```python
from build123d import *

# Parameters (mm, degrees)
BOSS_EXTRUDE1_DEPTH = 105
CUT_EXTRUDE1_REACH  = 238.485
SKETCH2_W           = 65
SKETCH2_H           = 15
CUT_EXTRUDE12_DEPTH = 281.35970199
CUT_EXTRUDE14_REACH = 239.237
FILLET1_R           = 10
FILLET2_R           = 10
FILLET3_R           = 10
FILLET4_R           = 2
CUT_EXTRUDE15_REACH = 239.237
SKETCH13_R          = 5
FILLET5_R           = 10


with BuildPart() as part:
    # Sketch1 → Boss-Extrude1 (new body)
    with BuildSketch(Plane.XY):
        Polygon((-125, -1.25), (125, -1.25), (126.885753532, -1.25), (146.885753532, 68.75), (200, 68.75), (200, 71.25), (145, 71.25), (125, 1.25), (-125, 1.25), align=None)
    extrude(amount=BOSS_EXTRUDE1_DEPTH)

    # Sketch2 → Cut-Extrude1 (cut, up to next)
    with BuildSketch(Plane(origin=(0, 1.25, 0), x_dir=(1, 0, 0), z_dir=(0, 1, 0)), mode=Mode.PRIVATE) as cut_extrude1_sk1:
        with Locations((-92.5, -52.5)):
            Rectangle(SKETCH2_W, SKETCH2_H)
    cut_extrude1_tool1 = extrude(cut_extrude1_sk1.sketch, amount=-CUT_EXTRUDE1_REACH, mode=Mode.PRIVATE) & part.part
    add(cut_extrude1_tool1.solids().sort_by_distance((-92.5, 1.25, 52.5))[0], mode=Mode.SUBTRACT)

    # Sketch11 → Cut-Extrude12 (cut, through all)
    with BuildSketch(Plane(origin=(125, 0, 0), x_dir=(0, 0, -1), z_dir=(1, 0, 0))):
        Polygon((0, 71.25), (0, 1.25), (-32.5, 68.75), (-32.5, 71.25), align=None)
        Polygon((-72.5, 68.75), (-72.5, 71.25), (-105, 71.25), (-105, 1.25), align=None)
    extrude(amount=CUT_EXTRUDE12_DEPTH, mode=Mode.SUBTRACT)

    # Sketch12 → Cut-Extrude14 (cut, up to next)
    with BuildSketch(Plane(origin=(0, 71.25, 0), x_dir=(1, 0, 0), z_dir=(0, 1, 0)), mode=Mode.PRIVATE) as cut_extrude14_sk1:
        Polygon((200, -62.5), (147.5, -72.5), (200, -72.5), align=None)
    cut_extrude14_tool1 = extrude(cut_extrude14_sk1.sketch, amount=-CUT_EXTRUDE14_REACH, mode=Mode.PRIVATE) & part.part
    # Sketch12 → Cut-Extrude14 (cut, up to next)
    with BuildSketch(Plane(origin=(0, 71.25, 0), x_dir=(1, 0, 0), z_dir=(0, 1, 0)), mode=Mode.PRIVATE) as cut_extrude14_sk2:
        Polygon((200, -32.5), (147.5, -32.5), (200, -42.5), align=None)
    cut_extrude14_tool2 = extrude(cut_extrude14_sk2.sketch, amount=-CUT_EXTRUDE14_REACH, mode=Mode.PRIVATE) & part.part
    add(cut_extrude14_tool1.solids().sort_by_distance((182.5, 71.25, 69.166667))[0], mode=Mode.SUBTRACT)
    add(cut_extrude14_tool2.solids().sort_by_distance((182.5, 71.25, 35.833333))[0], mode=Mode.SUBTRACT)

    # Fillet1
    fillet1_edges = [part.edges().sort_by_distance(p)[0] for p in [
        (200, 70, 42.5),
        (200, 70, 62.5),
    ]]
    fillet(fillet1_edges, radius=FILLET1_R)

    # Fillet2
    # the kernel refuses this fillet: 10 mm, written as the material it adds along each edge
    with BuildSketch(Plane(origin=(146.885753532, 68.75, 32.5), x_dir=(1, 0, 0), z_dir=(0, 0, 1))) as fillet2_piece_1_section:
        with BuildLine():
            CenterArc((FILLET2_R * 0.754301412754, -FILLET2_R), FILLET2_R, 90, 74.054604099)
            Line((-FILLET2_R * 0.207222534886, -FILLET2_R * 0.725278872103), (0, 0))
            Line((0, 0), (FILLET2_R * 0.754301412754, 0))
        make_face()
    fillet2_piece_1 = extrude(amount=40, mode=Mode.PRIVATE)
    fillet2_piece_1 = split(fillet2_piece_1, bisect_by=Plane(origin=(151.701250416, 67.179105295, 33.300238174), z_dir=(-0.18711210788999527, 0, 0.9823385664224747)), keep=Keep.TOP, mode=Mode.PRIVATE)
    fillet2_piece_1 = split(fillet2_piece_1, bisect_by=Plane(origin=(151.701250416, 67.179105295, 71.699761826), z_dir=(-0.18711210788999538, 0, -0.9823385664224747)), keep=Keep.TOP, mode=Mode.PRIVATE)
    add(fillet2_piece_1)
    # the kernel refuses this fillet: 10 mm, written as the material it takes off along each edge
    with BuildSketch(Plane(origin=(145, 71.25, 13.642464681), x_dir=(-0.27472112789737757, -0.9615239476408233, 0), z_dir=(0, 0, 1))) as fillet2_2_piece_1:
        with BuildLine():
            CenterArc((FILLET2_R * 0.754301412754, FILLET2_R), FILLET2_R, 195.945395901, 74.054604099)
            Line((-FILLET2_R * 0.207222534886, FILLET2_R * 0.725278872103), (0, 0))
            Line((0, 0), (FILLET2_R * 0.754301412754, 0))
        make_face()
    extrude(amount=77.715070638, mode=Mode.SUBTRACT)

    # Fillet3
    fillet3_edges = [part.edges().sort_by_distance(p)[0] for p in [
        (125, 1.25, 52.5),
    ]]
    fillet(fillet3_edges, radius=FILLET3_R)

    # Fillet4
    fillet4_edges = [part.edges().sort_by_distance(p)[0] for p in [
        (-60, 0, 45),
        (-60, 0, 60),
    ]]
    fillet(fillet4_edges, radius=FILLET4_R)

    # Sketch13 → Cut-Extrude15 (cut, up to next)
    with BuildSketch(Plane(origin=(0, 71.25, 0), x_dir=(1, 0, 0), z_dir=(0, 1, 0)), mode=Mode.PRIVATE) as cut_extrude15_sk1:
        with Locations(Location((190, -52.5, 0), (0, 0, 270))):
            Circle(SKETCH13_R)
    cut_extrude15_tool1 = extrude(cut_extrude15_sk1.sketch, amount=-CUT_EXTRUDE15_REACH, mode=Mode.PRIVATE) & part.part
    add(cut_extrude15_tool1.solids().sort_by_distance((190, 71.25, 52.5))[0], mode=Mode.SUBTRACT)

    # Fillet5
    fillet5_edges = [part.edges().sort_by_distance(p)[0] for p in [
        (-125, 0, 0),
        (-125, 0, 105),
    ]]
    fillet(fillet5_edges, radius=FILLET5_R)


solid = part.part
```
Could you check a few things on this model? Use its own coordinates, in mm. A direction names the side the tool comes from. Coordinates: 2 decimals unless noted, no trailing zeros. Write each loop counter-clockwise with the first axis right and the second up, starting at its lowest first coordinate (ties: lowest second). Pieces come first, ordered by that corner, then holes. Notation, with made-up numbers: (62, -28.75) - (99, -28.75) arc R21 cw to (99, -15.75) - close; hole circle Ø8 at (31, 87.5). An arc over 180 degrees is marked (long way). Use a Markdown table: item, result.
Q1. I'm going to push flat-ended pins straight in: pin 1 Ø1 at (y, z) = (31, 74) entering from -X; pin 2 Ø6 at (y, z) = (46, 65.5) entering from +X; pin 3 Ø2 at (y, z) = (0, 54) entering from -X; pin 4 Ø9 at (x, z) = (190, 52.5) entering from -Y. Where does each tip first touch, or does it pass through?
Geometry check:
| item | result |
|---|---|
| pin 1 | stops at x = 133.36 |
| pin 2 | stops at x = 141.24 |
| pin 3 | stops at x = -60 |
| pin 4 | passes through |
Q2. Thinking about a two-plate mould opening in X: for faces 1 (the flat face through (-1, -1.25, 52)), 2 (the cylindrical face through (194.957, 70.018, 51.849)), 3 (the cylindrical face through (148.48, 66.79, 52.22)), which applies, +X half, -X half, draft (parallel to the pull), parting line (faces both ways), or undercut?
Geometry check:
| item | result |
|---|---|
| face 1 | draft |
| face 2 | undercut |
| face 3 | +X half |
Q3. Please list where these lines run through material, in increasing order: L1, parallel to Y at x = -110, z = 75; L2, parallel to X at y = 70.05, z = 52.5.
Geometry check:
| item | result |
|---|---|
| L1 | y = -1.25 to 1.25 |
| L2 | x = 147.79 to 185, 195 to 200 |
Q4. Which directions (+Z, -Z, +X, -X, +Y, -Y) give clear straight access to the entire face, cutting with the end or side of a thin tool? Please do faces 4 (the flat face through (172, 68.75, 52)), 5 (the flat face through (-2, 1.25, 52)), 6 (the flat face through (169.996, 69.818, 68.215)).
Geometry check:
| item | result |
|---|---|
| face 4 | +Z, -Z, +X, -Y |
| face 5 | +Z, -Z, -X, +Y |
| face 6 | +Z, +X, +Y, -Y |
Q5. Imagine slicing it at A-A (x = -83.5). List the corners of the cut face in (y, z) for me.
Geometry check:
| item | result |
|---|---|
| outline | (-1.25, 0) - (1.25, 0) - (1.25, 45) - (-1.25, 45) - close; (-1.25, 60) - (1.25, 60) - (1.25, 105) - (-1.25, 105) - close |
Q6. Imagine slicing it at C-C (y = 34.5). List the corners of the cut face in (x, z) for me.
Geometry check:
| item | result |
|---|---|
| outline | (134.5, 16.01) - (137.1, 16.01) - (137.1, 88.99) - (134.5, 88.99) - close |
Q7. Imagine slicing it at B-B (z = 18.5). List the corners of the cut face in (x, y) for me, and give its area (3 significant figures).
Geometry check:
| item | result |
|---|---|
| outline | (-125, -1.25) - (126.89, -1.25) - (138.58, 39.67) - (135.98, 39.67) - (127.07, 8.5) arc R10 cw to (117.46, 1.25) - (-125, 1.25) - close |
| area | 741 mm2 |
Q8. Imagine slicing it at D-D (x = 11). List the corners of the cut face in (y, z) for me, and give its area (4 significant figures).
Geometry check:
| item | result |
|---|---|
| outline | (-1.25, 0) - (1.25, 0) - (1.25, 105) - (-1.25, 105) - close |
| area | 262.5 mm2 |
